Verification items for the finished model (mm, model axes). Face numbers are marked on the shaded views. A direction names the side the tool comes from. Round coordinates to 2 decimals unless told otherwise and drop trailing zeros. Write each loop counter-clockwise with the first axis right and the second up, starting at its lowest first coordinate (ties: lowest second). Pieces come first, ordered by that corner, then holes. Notation, with made-up numbers: (10.5, 30.5) -> (67.5, 30.5) arc R16 ccw to (67.5, 53.5) -> close; hole circle Ø1 at (71, -38). An arc over 180 degrees is marked (long way). Answer as a JSON object with one key per item and string values. Group by question number.
(1) Gauge pin test, flat ends, axial feed: pin 1 Ø1.5 at (x, z) = (5, -0.5) entering from +Y; pin 2 Ø1.5 at (y, z) = (-1, 1) entering from +X. Record the tip position at first contact, or that the pin passes through.
(2) Sectioned sample at A-A on x = 0.25. Record the cut outline in (y, z).
(3) Draft check along Z on the marked faces 3, 4 and 5. Enter one of: released by +Z, released by -Z, zero draft, split by the parting line, or undercut.
(4) Set-up check for the marked faces 1 and 2: record each of +Z, -Z, +X, -X, +Y, -Y from which the full face is reachable in a straight line by a thin tool's end or side.
(5) Scan lines: L1, parallel to X at y = -0.15, z = -1.15; L2, parallel to Z at x = 3, y = 0.05; L3, parallel to Y at x = 3.5, z = -0.9. Record each from-to range of solid material in increasing order. Write a range as from..to.
```python
from build123d import *

# Parameters (mm, degrees)
CUT_EXTRUDE1_DEPTH = 1


with BuildPart() as part:
    # Sketch1 → Revolve1 (revolve)
    with BuildSketch(Plane.XY):
        Polygon((-2, 0), (-2, 1.3125), (-1.8125, 1.5), (0, 1.5), (0, 1), (5.7545, 1), (6, 0.7545), (6, 0), align=None)
    revolve(axis=Axis((6, 0, 0), (-1, 0, 0)))

    # Sketch2 → Cut-Revolve1 (revolve, cut)
    with BuildSketch(Plane.XY):
        Polygon((-2, 0), (-2, 0.9), (-1.85, 0.75), (-1, 0.75), (-0.6, 0), align=None)
    revolve(axis=Axis((-0.6, 0, 0), (-1, 0, 0)), mode=Mode.SUBTRACT)

    # Sketch3 → Cut-Extrude1 (cut)
    with BuildSketch(Plane(origin=(-2, 0, 0), x_dir=(0, 0, -1), z_dir=(1, 0, 0))):
        Polygon((-0.75, -0.433012702), (0, -0.866025404), (0.75, -0.433012702), (0.75, 0.433012702), (0, 0.866025404), (-0.75, 0.433012702), align=None)
    extrude(amount=CUT_EXTRUDE1_DEPTH, mode=Mode.SUBTRACT)


solid = part.part
```
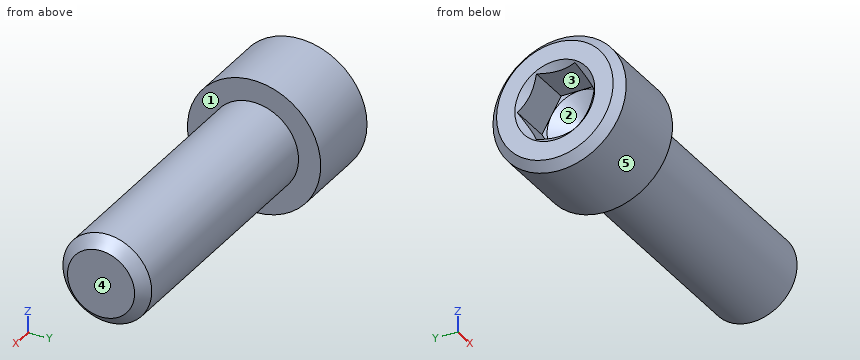
Computed values:
{
 "1": {"pin 1": "y = 1", "pin 2": "x = 6"},
 "2": {"outline": "circle Ø2 at (0, 0)"},
 "3": {"face 3": "undercut", "face 4": "zero draft", "face 5": "split by the parting line"},
 "4": {"face 1": "+X", "face 2": "-X"},
 "5": {"L1": "-2..0", "L2": "-1..1", "L3": "-0.44..0.44"}
}
